Autodesk Inventor part; units mm, degrees
ref_plane "Work Plane1" through (204.9, -63.9793, -16.6497) normal (-0.5735764, 0, -0.819152) x (-0.819152, 0, 0.5735764)
ref_plane "YZ Plane" through (0, 0, 0) normal (1, 0, 0) x (0, 1, 0)
ref_plane "XZ Plane" through (0, 0, 0) normal (0, 1, 0) x (-1, 0, 0)
sketch "Sketch1" plane through (0, 0, 0) normal (0, 0, 1) x (1, 0, 0)
  line L0 (-10.4542, 14.6019) -> (210.2083, 14.6019)
  line L1 (216.5583, 8.2519) -> (216.5583, -98.1106)
  line L2 (210.2083, -104.4606) -> (-10.4542, -104.4606)
  line L3 (-16.8042, -98.1106) -> (-16.8042, 8.2519)
  line L4 (99.877, 12.2207) -> (-10.4542, 12.2207)
  line L5 (-14.423, 8.2519) -> (-14.423, -44.9293)
  line L6 (99.877, 12.2207) -> (210.2083, 12.2207)
  line L7 (214.177, 8.2519) -> (214.177, -44.9293)
  line L8 (99.877, -102.0793) -> (210.2083, -102.0793)
  line L9 (214.177, -98.1106) -> (214.177, -44.9293)
  line L10 (99.877, -102.0793) -> (-10.4542, -102.0793)
  line L11 (-14.423, -98.1106) -> (-14.423, -44.9293)
  arc A0 (-10.4542, 14.6019) -> (-16.8042, 8.2519) centre (-10.4542, 8.2519) ccw
  arc A1 (216.5583, 8.2519) -> (210.2083, 14.6019) centre (210.2083, 8.2519) ccw
  arc A2 (210.2083, -104.4606) -> (216.5583, -98.1106) centre (210.2083, -98.1106) ccw
  arc A3 (-16.8042, -98.1106) -> (-10.4542, -104.4606) centre (-10.4542, -98.1106) ccw
  arc A4 (-10.4542, 12.2207) -> (-14.423, 8.2519) centre (-10.4542, 8.2519) ccw
  arc A5 (214.177, 8.2519) -> (210.2083, 12.2207) centre (210.2083, 8.2519) ccw
  arc A6 (210.2083, -102.0793) -> (214.177, -98.1106) centre (210.2083, -98.1106) ccw
  arc A7 (-14.423, -98.1106) -> (-10.4542, -102.0793) centre (-10.4542, -98.1106) ccw
  point P0 (0, 0)
  point P1 (-16.8042, 14.6019)
  point P2 (216.5583, -104.4606)
  point P3 (216.5583, 14.6019)
  point P4 (-16.8042, -104.4606)
  dimension "d0" = 233.3625
  dimension "d1" = 119.0625
  dimension "d9" = 6.35
  dimension "d10" = 3.9688
extrude "Extrusion1" add sketch "Sketch1" along normal blind 2.3813 contours L0 A1 L1 A2 L2 A3 L3 A0 | L6 A5 L7 L9 A6 L8 L10 A7 L11 L5 A4 L4
sketch "Sketch2" plane through (0, 0, 2.3813) normal (0, 0, 1) x (1, 0, 0)
  line L0 (210.2083, 14.6019) -> (-10.4542, 14.6019)
  arc A0 (-10.4542, 14.6019) -> (-16.8042, 8.2519) centre (-10.4542, 8.2519) ccw
  line L1 (-16.8042, 8.2519) -> (-16.8042, -98.1106)
  arc A1 (-16.8042, -98.1106) -> (-10.4542, -104.4606) centre (-10.4542, -98.1106) ccw
  line L2 (-10.4542, -104.4606) -> (210.2083, -104.4606)
  arc A2 (210.2083, -104.4606) -> (216.5583, -98.1106) centre (210.2083, -98.1106) ccw
  line L3 (216.5583, -98.1106) -> (216.5583, 8.2519)
  arc A3 (216.5583, 8.2519) -> (210.2083, 14.6019) centre (210.2083, 8.2519) ccw
  line L4 (99.877, 12.2207) -> (-10.4542, 12.2207)
  line L5 (-14.423, 8.2519) -> (-14.423, -44.9293)
  line L6 (99.877, -102.0793) -> (-10.4542, -102.0793)
  line L7 (-14.423, -98.1106) -> (-14.423, -44.9293)
  line L8 (99.877, -102.0793) -> (210.2083, -102.0793)
  line L9 (214.177, -98.1106) -> (214.177, -44.9293)
  line L10 (99.877, 12.2207) -> (210.2083, 12.2207)
  line L11 (214.177, 8.2519) -> (214.177, -44.9293)
  arc A4 (-10.4542, 12.2207) -> (-14.423, 8.2519) centre (-10.4542, 8.2519) ccw
  arc A5 (214.177, 8.2519) -> (210.2083, 12.2207) centre (210.2083, 8.2519) ccw
  arc A6 (210.2083, -102.0793) -> (214.177, -98.1106) centre (210.2083, -98.1106) ccw
  arc A7 (-14.423, -98.1106) -> (-10.4542, -102.0793) centre (-10.4542, -98.1106) ccw
  point P0 (0, 0)
  dimension "d15" = 3.9688
extrude "Extrusion2" add sketch "Sketch2" along normal blind 2.3813
sketch "Sketch3" plane through (0, 0, 4.7625) normal (0, 0, 1) x (1, 0, 0)
  arc A0 (-10.4542, 12.2207) -> (-14.423, 8.2519) centre (-10.4542, 8.2519) ccw
  arc A1 (214.177, 8.2519) -> (210.2083, 12.2207) centre (210.2083, 8.2519) ccw
  line L0 (214.177, 8.2519) -> (214.177, -98.1106)
  arc A2 (210.2083, -102.0793) -> (214.177, -98.1106) centre (210.2083, -98.1106) ccw
  line L1 (210.2083, -102.0793) -> (-10.4542, -102.0793)
  arc A3 (-14.423, -98.1106) -> (-10.4542, -102.0793) centre (-10.4542, -98.1106) ccw
  line L2 (-14.423, -98.1106) -> (-14.423, 8.2519)
  arc A4 (-10.4542, 14.6019) -> (-16.8042, 8.2519) centre (-10.4542, 8.2519) ccw
  line L3 (-16.8042, 8.2519) -> (-16.8042, -98.1106)
  arc A5 (-16.8042, -98.1106) -> (-10.4542, -104.4606) centre (-10.4542, -98.1106) ccw
  line L4 (-10.4542, -104.4606) -> (210.2083, -104.4606)
  arc A6 (210.2083, -104.4606) -> (216.5583, -98.1106) centre (210.2083, -98.1106) ccw
  line L5 (216.5583, -98.1106) -> (216.5583, 8.2519)
  arc A7 (216.5583, 8.2519) -> (210.2083, 14.6019) centre (210.2083, 8.2519) ccw
  line L6 (214.177, -44.9293) -> (214.177, -41.7543)
  line L7 (214.177, -41.7543) -> (216.5583, -41.7543)
  line L8 (216.5583, -41.7543) -> (216.5583, -44.9293)
  line L9 (216.5583, -44.9293) -> (216.5583, -48.1043)
  line L10 (216.5583, -48.1043) -> (214.177, -48.1043)
  line L11 (214.177, -48.1043) -> (214.177, -44.9293)
  line L12 (-14.423, -44.9293) -> (-14.423, -41.7543)
  line L13 (-14.423, -41.7543) -> (-16.8042, -41.7543)
  line L14 (-16.8042, -41.7543) -> (-16.8042, -44.9293)
  line L15 (-16.8042, -44.9293) -> (-16.8042, -48.1043)
  line L16 (-16.8042, -48.1043) -> (-14.423, -48.1043)
  line L17 (-14.423, -48.1043) -> (-14.423, -44.9293)
  line L18 (-10.4542, 14.6019) -> (25.1058, 14.6019)
  line L19 (25.1058, 14.6019) -> (25.1058, 12.2207)
  line L20 (37.8058, 14.6019) -> (37.8058, 12.2207)
  line L21 (-10.4542, 12.2207) -> (25.1058, 12.2207)
  line L22 (37.8058, 12.2207) -> (210.2083, 12.2207)
  line L23 (37.8058, 14.6019) -> (210.2083, 14.6019)
  point P0 (0, 0)
  dimension "d18" = 3.175
  dimension "d19" = 3.175
  dimension "d20" = 3.175
  dimension "d21" = 3.175
  dimension "d93" = 35.56
  dimension "d94" = 12.7
extrude "Extrusion3" add sketch "Sketch3" along normal blind 10.3188 contours A0 L2 L13 L3 A4 L18 L19 L21 | L2 A3 L1 A2 L0 L10 L5 A6 L4 A5 L3 L16
sketch "Sketch4" plane through (0, 0, 15.0813) normal (0, 0, 1) x (1, 0, 0)
  line L0 (214.177, -41.7543) -> (216.5583, -41.7543)
  line L1 (216.5583, -41.7543) -> (216.5583, -48.1043)
  line L2 (216.5583, -48.1043) -> (214.177, -48.1043)
  line L3 (214.177, -48.1043) -> (214.177, -41.7543)
  line L4 (-16.8042, -41.7543) -> (-14.423, -41.7543)
  line L5 (-14.423, -41.7543) -> (-14.423, -48.1043)
  line L6 (-14.423, -48.1043) -> (-16.8042, -48.1043)
  line L7 (-16.8042, -48.1043) -> (-16.8042, -41.7543)
  point P0 (0, 0)
  dimension "d24" = 2.3813
  dimension "d25" = 6.35
  dimension "d26" = 2.3813
  dimension "d27" = 6.35
extrude "Extrusion4" add sketch "Sketch4" against normal blind 7.9375
sketch "Sketch5" plane through (0, 0, 0) normal (0, 0, -1) x (-1, 0, 0)
  arc A0 (-210.2083, 14.6019) -> (-216.5583, 8.2519) centre (-210.2083, 8.2519) ccw
  line L0 (-210.2083, 8.2519) -> (-99.877, 8.2519)
  line L1 (-99.877, 8.2519) -> (-99.877, -44.9293)
  line L2 (-99.877, -44.9293) -> (-210.2083, -44.9293)
  line L3 (-210.2083, -44.9293) -> (-210.2083, 8.2519)
  point P0 (0, 0)
hole "Hole1" at (99.877, -44.9293, 0) direction (0, 0, 1) diameter 19.05 end through all
sketch "Sketch6" plane through (0, 0, 0) normal (0, 0, -1) x (-1, 0, 0)
  line L0 (-216.5583, 8.2519) -> (-216.5583, -98.1106)
  line L1 (-216.5583, -25.8793) -> (-216.5583, -63.9793)
  line L2 (-216.5583, -63.9793) -> (-170.0509, -63.9793)
  line L3 (-170.0509, -63.9793) -> (-170.0509, -25.8793)
  line L4 (-170.0509, -25.8793) -> (-216.5583, -25.8793)
  point P0 (0, 0)
  dimension "d39" = 38.1
  dimension "d43" = 46.5074
extrude "Extrusion6" add sketch "Sketch6" along normal blind 38.1
sketch "Sketch8" plane through (170.0509, -25.8793, 0) normal (0, 1, 0) x (1, 0, 0)
  line L0 (46.5074, 0) -> (13.7658, 46.7599)
  point P0 (46.5074, 38.1)
  point P1 (0, 38.1)
  point P2 (-170.0509, 0)
split body "Split1" sketch "Sketch8" result one side removed curves L0 removed pieces at (208.0752, -38.5793, -12.9868)
sketch "Sketch9" plane through (170.0509, -25.8793, 0) normal (0, 1, 0) x (1, 0, 0)
  line L0 (0, 0) -> (64.0379, 44.8398)
  line L1 (0, 0) -> (78.1758, 0) construction
  line L2 (0, 0) -> (0, 38.1)
  point P0 (-170.0509, 0)
  dimension "d48" = 35
split body "Split2" sketch "Sketch9" result one side removed curves L2 L0 removed pieces at (170.5509, -51.2793, -12.7)
ref_plane "Work Plane1" through (204.9, -63.9793, -16.6497) normal (-0.5735764, 0, -0.819152) x (-0.819152, 0, 0.5735764)
sketch "Sketch10" plane through (204.9, -63.9793, -16.6497) normal (-0.5735764, 0, -0.819152) x (-0.819152, 0, 0.5735764)
  line L0 (0, 38.1) -> (38.0966, 38.1)
  line L1 (0, 0) -> (0, 38.1)
  line L2 (38.0966, 0) -> (0, 0)
  line L3 (38.0966, 38.1) -> (38.0966, 0)
  line L4 (19.0483, 38.1) -> (19.0483, 28.575)
  line L5 (19.0483, 0) -> (19.0483, 9.525)
  point P0 (177.3942, 63.9793)
  dimension "d50" = 9.525
  dimension "d51" = 9.525
hole "Hole2" at (189.2966, -35.4043, -5.724) at (189.2966, -54.4543, -5.724) direction (0.5735764, 0, 0.819152) diameter 13.4938 end through all
sketch "Sketch11" plane through (204.9, -63.9793, -16.6497) normal (-0.5735764, 0, -0.819152) x (-0.819152, 0, 0.5735764)
  line L0 (0, 38.1) -> (38.0966, 38.1)
  line L1 (0, 0) -> (0, 38.1)
  line L2 (38.0966, 0) -> (0, 0)
  line L3 (38.0966, 38.1) -> (38.0966, 0)
  line L4 (19.0483, 38.1) -> (19.0483, 28.575)
  line L5 (19.0483, 0) -> (19.0483, 9.525)
  point P0 (177.3942, 63.9793)
  dimension "d59" = 9.525
  dimension "d60" = 9.525
hole "Hole3" at (189.2966, -35.4043, -5.724) at (189.2966, -54.4543, -5.724) direction (-0.5735764, 0, -0.819152) diameter 8.3312 end through all
sketch "Sketch12" plane through (0, 0, 4.7625) normal (0, 0, 1) x (1, 0, 0)
  line L0 (216.5583, -41.7543) -> (214.177, -41.7543)
  line L1 (214.177, 8.2519) -> (214.177, -48.1043)
  line L2 (216.5583, -41.7543) -> (214.177, -41.7543)
  line L3 (214.177, -41.7543) -> (214.177, -48.1043)
  line L4 (214.177, -48.1043) -> (216.5583, -48.1043)
  line L5 (216.5583, -48.1043) -> (216.5583, -41.7543)
  point P0 (0, 0)
extrude "Extrusion7" add sketch "Sketch12" along normal blind 2.3876
sketch "Sketch13" plane through (0, 0, 4.7625) normal (0, 0, 1) x (1, 0, 0)
  line L0 (-14.423, -41.7543) -> (-16.8042, -41.7543)
  line L1 (-16.8042, -41.7543) -> (-16.8042, -48.1043)
  line L2 (-14.423, -41.7543) -> (-16.8042, -41.7543)
  line L3 (-16.8042, -41.7543) -> (-16.8042, -48.1043)
  line L4 (-16.8042, -48.1043) -> (-14.423, -48.1043)
  line L5 (-14.423, -48.1043) -> (-14.423, -41.7543)
  point P0 (0, 0)
extrude "Extrusion8" add sketch "Sketch13" along normal blind 2.3876
sketch "Sketch16" plane through (0, 0, 0) normal (0, 0, -1) x (-1, 0, 0)
  arc A0 (-210.2083, 14.6019) -> (-216.5583, 8.2519) centre (-210.2083, 8.2519) ccw
  arc A1 (-216.5583, -98.1106) -> (-210.2083, -104.4606) centre (-210.2083, -98.1106) ccw
  arc A2 (10.4542, -104.4606) -> (16.8042, -98.1106) centre (10.4542, -98.1106) ccw
  arc A3 (16.8042, 8.2519) -> (10.4542, 14.6019) centre (10.4542, 8.2519) ccw
  point P0 (0, 0)
hole "Hole6" at (210.2083, 8.2519, 0) at (-10.4542, 8.2519, 0) at (-10.4542, -98.1106, 0) at (210.2083, -98.1106, 0) direction (0, 0, 1) diameter 3.175 end through all
sketch "Sketch17" plane through (0, 0, 4.7625) normal (0, 0, 1) x (1, 0, 0)
  line L0 (214.177, -41.7543) -> (216.5583, -41.7543)
  line L1 (216.5583, -41.7543) -> (216.5583, 8.2519)
  arc A0 (216.5583, 8.2519) -> (210.2083, 14.6019) centre (210.2083, 8.2519) ccw
  line L2 (210.2083, 14.6019) -> (25.1058, 14.6019)
  line L3 (25.1058, 12.2207) -> (210.2083, 12.2207)
  arc A1 (214.177, 8.2519) -> (210.2083, 12.2207) centre (210.2083, 8.2519) ccw
  line L4 (214.177, 8.2519) -> (214.177, -41.7543)
  line L5 (25.1058, 14.6019) -> (37.8058, 14.6019)
  line L6 (37.8058, 14.6019) -> (37.8058, 12.2207)
  point P0 (0, 0)
  dimension "d95" = 12.7
extrude "Extrusion9" add sketch "Sketch17" along normal blind 10.3124
sketch "Sketch18" plane through (0, 0, 4.7625) normal (0, 0, 1) x (1, 0, 0)
  line L0 (37.8058, 12.2207) -> (37.8058, 14.6019)
  line L1 (37.8058, 14.6019) -> (25.1058, 14.6019)
  line L2 (25.1058, 14.6019) -> (25.1058, 12.2207)
  line L3 (25.1058, 12.2207) -> (37.8058, 12.2207)
  point P0 (0, 0)
extrude "Extrusion10" add sketch "Sketch18" along normal blind 2.6924
properties part number "Slave Tablet Enclosure"
Can you work these out from the model? Positions are in its coordinate system, mm. A direction names the side the tool comes from. Give positions to 0.01 mm unless a question says otherwise; leave off trailing zeros. Loops run counter-clockwise (first coordinate to the right, second up) from the corner with the lowest first, then second, coordinate; pieces in that order, holes last. Notation, with made-up numbers: M 81.25,29.5 L 136.25,29.5 A10 cw 136.25,37.5 Z; hole C 59.25,18.25 d11. An arc over 180 degrees is marked long. Use one line per item in the form item = value. Start each with the question number.
(1) Thinking about a two-plate mould opening in Z: for faces 4 (the flat face through (127, 14, 15.075)), 5 (the cylindrical face through (214.65, 12.79, 7.43)), 6 (the flat face through (192.904, -35.499, -8.25)), which applies, released by +Z, released by -Z, zero draft, split by the parting line, or undercut?
(2) On a 3-axis mill with a long thin cutter (end or side, diameter ignored), from which of +Z, -Z, +X, -X, +Y, -Y can I reach the whole of each face in a straight line? I mean faces 1 (the flat face through (198, -25.879, -6)), 2 (the flat face through (194, -63.979, -6)), 3 (the flat face through (98, 12.221, 9)). Say none if no direction works.
(3) I want a section at B-B, the plane x = 81.5. Write out the boundary of the cut face in (y, z), and give its area (3 significant figures).
(4) I want a section at A-A, the plane y = -19.5. Write out the boundary of the cut face in (x, z), and give its area (3 significant figures).
(5) I want a section at C-C, the plane z = 4.5. Write out the boundary of the cut face in (x, y), and give its area (3 significant figures).
(6) Please list where these lines run through material, in increasing order: line 1 (Y direction, x = 119.5, z = 8); line 2 (X direction, y = -66, z = 7); line 3 (Z direction, x = 42, y = -90).
(7) I want a section at D-D, the plane z = -19.5. Write out the boundary of the cut face in (x, y).
(8) I'm going to push flat-ended pins straight in: P1, Ø17, axis at x = 99.88, y = -44.93, coming from the -Z side; P2, Ø1.9, axis at x = 31.5, y = 13.5, coming from the +Z side; P3, Ø1.5, axis at y = -58.5, z = -3, coming from the +X side; P4, Ø1, axis at x = 47, y = -29, coming from the -Z side. Where does each tip first touch, or does it pass through?
Worked out:
q1.face_4 = released by +Z
q1.face_5 = zero draft
q1.face_6 = undercut
q2.face_1 = -Z, +X, -X, +Y
q2.face_2 = -Z, +X, -X, -Y
q2.face_3 = +Z
q3.outline = M -104.46,0 L 14.6,0 L 14.6,15.07 L 12.22,15.07 L 12.22,2.38 L -102.08,2.38 L -102.08,15.08 L -104.46,15.08 Z
q3.area = 344 mm²
q4.outline = M -16.8,0 L 216.56,0 L 216.56,15.07 L 214.18,15.07 L 214.18,2.38 L -14.42,2.38 L -14.42,15.08 L -16.8,15.08 Z
q4.area = 616 mm²
q5.outline = M -16.8,-98.11 A6.35 ccw -10.45,-104.46 L 210.21,-104.46 A6.35 ccw 216.56,-98.11 L 216.56,8.25 A6.35 ccw 210.21,14.6 L -10.45,14.6 A6.35 ccw -16.8,8.25 Z; hole M -14.42,-98.11 A3.97 ccw -10.45,-102.08 L 210.21,-102.08 A3.97 ccw 214.18,-98.11 L 214.18,8.25 A3.97 ccw 210.21,12.22 L -10.45,12.22 A3.97 ccw -14.42,8.25 Z
q5.area = 1,630 mm²
q6.line_1 = -104.46 to -102.08, 12.22 to 14.6
q6.line_2 = -16.8 to -14.42, 214.18 to 216.56
q6.line_3 = 0 to 2.38
q7.outline = M 197.9,-63.98 L 202.9,-63.98 L 202.9,-25.88 L 197.9,-25.88 Z
q8.P1 = through
q8.P2 = 7.45
q8.P3 = 214.98
q8.P4 = 0
